Autodesk Inventor part; units mm, degrees
ref_plane "YZ Plane" through (0, 0, 0) normal (1, 0, 0) x (0, 1, 0)
ref_plane "XZ Plane" through (0, 0, 0) normal (0, 1, 0) x (-1, 0, 0)
ref_plane "XY Plane" through (0, 0, 0) normal (0, 0, 1) x (1, 0, 0)
ref_plane "РабПлоскость1" through (-34.9448, 28.465, -130.3508) normal (0, 0, 1) x (1, 0, 0)
ref_plane "РабПлоскость2" through (-162.802, 331.465, 111.3492) normal (0, 0, 1) x (1, 0, 0)
sketch "Эскиз1" plane through (-34.9448, 28.465, -130.3508) normal (0, 0, 1) x (1, 0, 0)
  line L0 (0, 3.6904) -> (-12.8571, 3.6904) construction
  line L1 (0, 3.6904) -> (0, 9.6905)
  line L2 (-12.8571, 9.6905) -> (0, 9.6905)
  line L3 (-12.8571, 3.6904) -> (-12.8571, 9.6905)
  line L4 (25.7143, 3.6904) -> (12.8571, 3.6904) construction
  line L5 (25.7143, 3.6904) -> (25.7143, 9.6905)
  line L6 (12.8571, 9.6905) -> (25.7143, 9.6905)
  line L7 (12.8571, 3.6904) -> (12.8571, 9.6905)
  line L8 (51.4286, 3.6904) -> (38.5714, 3.6904) construction
  line L9 (51.4286, 3.6904) -> (51.4286, 9.6905)
  line L10 (38.5714, 9.6905) -> (51.4286, 9.6905)
  line L11 (38.5714, 3.6904) -> (38.5714, 9.6905)
  line L12 (77.1429, 3.6904) -> (64.2857, 3.6904) construction
  line L13 (77.1429, 3.6904) -> (77.1429, 9.6905)
  line L14 (64.2857, 9.6905) -> (77.1429, 9.6905)
  line L15 (64.2857, 3.6904) -> (64.2857, 9.6905)
  line L16 (0, 3.6904) -> (12.8571, 3.6904)
  line L17 (25.7143, 3.6904) -> (38.5714, 3.6904)
  line L18 (51.4286, 3.6904) -> (64.2857, 3.6904)
  line L19 (-12.8571, 3.6904) -> (-12.8571, -50.3096)
  line L20 (-9.8571, -53.3096) -> (-4.7353, -53.3096)
  line L21 (77.1429, 3.6904) -> (77.1429, -50.3096)
  line L22 (74.1429, -53.3096) -> (69.021, -53.3096)
  line L23 (-1.8571, -53.3096) -> (66.1429, -53.3096) construction
  arc A0 (-1.7452, -56.0663) -> (66.0309, -56.0663) centre (32.1429, -53.3096) ccw
  arc A1 (-1.7452, -56.0663) -> (-4.7353, -53.3096) centre (-4.7353, -56.3096) ccw
  arc A2 (69.021, -53.3096) -> (66.0309, -56.0663) centre (69.021, -56.3096) ccw
  arc A3 (74.1429, -53.3096) -> (77.1429, -50.3096) centre (74.1429, -50.3096) ccw
  arc A4 (-12.8571, -50.3096) -> (-9.8571, -53.3096) centre (-9.8571, -50.3096) ccw
  circle A5 centre (32.1429, -53.3095) radius 2.375
  point P0 (34.9448, -28.465)
  point P1 (77.1429, -53.3096)
  dimension "d0" = 57
  dimension "d1" = 34
  dimension "d2" = 3
  dimension "d3" = 6
  dimension "d14" = 4.75
extrude "Выдавливание1" add sketch "Эскиз1" along normal blind 6
sketch "Эскиз2" plane through (-34.9448, 28.465, -130.3508) normal (0, 0, -1) x (-1, 0, 0)
  line L0 (-4.9286, 3.6904) -> (-4.9286, -2.6596)
  line L1 (-4.9286, -2.6596) -> (-3.6786, -2.6596)
  line L2 (-3.6786, -2.6596) -> (-3.6786, -4.9596)
  line L3 (-3.6786, -4.9596) -> (-4.9286, -4.9596)
  line L4 (-4.9286, -4.9596) -> (-4.9286, -11.3096)
  line L5 (-4.9286, -11.3096) -> (-7.9286, -11.3096)
  line L6 (-7.9286, -11.3096) -> (-7.9286, -4.9596)
  line L7 (-7.9286, -4.9596) -> (-9.1786, -4.9596)
  line L8 (-9.1786, -4.9596) -> (-9.1786, -2.6596)
  line L9 (-9.1786, -2.6596) -> (-7.9286, -2.6596)
  line L10 (-7.9286, -2.6596) -> (-7.9286, 3.6904)
  line L11 (-56.3571, 3.6904) -> (-59.3571, 3.6904)
  line L12 (-56.3571, 3.6904) -> (-56.3571, -2.6596)
  line L13 (-56.3571, -2.6596) -> (-55.1071, -2.6596)
  line L14 (-55.1071, -2.6596) -> (-55.1071, -4.9596)
  line L15 (-55.1071, -4.9596) -> (-56.3571, -4.9596)
  line L16 (-56.3571, -4.9596) -> (-56.3571, -11.3096)
  line L17 (-56.3571, -11.3096) -> (-59.3571, -11.3096)
  line L18 (-59.3571, -11.3096) -> (-59.3571, -4.9596)
  line L19 (-59.3571, -4.9596) -> (-60.6071, -4.9596)
  line L20 (-60.6071, -4.9596) -> (-60.6071, -2.6596)
  line L21 (-60.6071, -2.6596) -> (-59.3571, -2.6596)
  line L22 (-59.3571, -2.6596) -> (-59.3571, 3.6904)
  line L23 (-56.3571, 3.6904) -> (-59.3571, 3.6904)
  line L24 (-4.9286, 3.6904) -> (-7.9286, 3.6904)
  point P0 (-34.9448, -28.465)
  point P1 (-6.4286, 0)
  dimension "d9" = 5.5
  dimension "d10" = 2.3
  dimension "d11" = 15
extrude "Выдавливание2" cut sketch "Эскиз2" against normal blind 6
equation "\"d4\" = d3"
equation "\"d12\" = d3"
properties part number "Korpus 4"
Design review of the part built by this model. Coordinates are the model's own, in mm. A direction names the side the tool comes from. Give positions to 0.01 mm unless a question says otherwise; leave off trailing zeros. Loops run counter-clockwise (first coordinate to the right, second up) from the corner with the lowest first, then second, coordinate; pieces in that order, holes last. Notation, with made-up numbers: (53.5, 25.25) - (81.5, 25.25) arc R16 cw to (81.5, 42.25) - close; hole circle Ø1 at (-40, -1). An arc over 180 degrees is marked (long way). Use CSV: the item, a comma, the result in double quotes. Start each with the question number.
1. Draft analysis for pull direction X (two halves, no side actions). For faces 3 (the flat face through (-27.016, 20, -127)), 4 (the cylindrical face through (-37.67, -25.62, -127.39)), 5 (the cylindrical face through (32.02, -25.66, -127.39)), 6 (the flat face through (37, -24.845, -127)), state which applies: released by +X, released by -X, zero draft, split by the parting line, or undercut.
2. Wall thickness on L1, parallel to X at y = -27.5, z = -126.15; L2, parallel to Y at x = 35, z = -125.9; L3, parallel to X at y = -22, z = -128.2: over which ranges is each line inside the solid? List them lowest first.
3. Insertion check: P1, Ø3, axis at x = 0, z = -126, coming from the +Y side; P2, Ø1.5, axis at y = -36, z = -126, coming from the -X side. Each pin has a flat end and moves straight along its axis. Give the tip position at first contact, or say it passes through.
4. Machinability: for faces 1 (the flat face through (-25, 32.155, -127)), 2 (the flat face through (-47.802, 9, -127)), which of the approach directions +Z, -Z, +X, -X, +Y, -Y give a long, thin tool a straight path to every point of the face, cutting with its end or side? Answer none if there is none.
5. Add section A-A (y = 29). State the section outline as (x, z) points, plus the area to 3 significant figures.
6. Add section B-B (y = -41). State the section outline as (x, z) points, plus the area to 3 significant figures.
Results found:
1,face 3,"undercut"
1,face 4,"released by -X"
1,face 5,"released by +X"
1,face 6,"zero draft"
2,L1,"x = -36.7 to 31.1"
2,L2,"y = -24.84 to 38.16"
2,L3,"x = -47.8 to 42.19"
3,P1,"stops at y = 32.16"
3,P2,"stops at x = -35.17"
4,face 1,"+Z, -Z, +Y"
4,face 2,"+Z, -Z, -X, +Y, -Y"
5,outline,"(-47.8, -130.35) - (-30.02, -130.35) - (-30.02, -124.35) - (-47.8, -124.35) - close; (-27.02, -130.35) - (21.41, -130.35) - (21.41, -124.35) - (-27.02, -124.35) - close; (24.41, -130.35) - (42.2, -130.35) - (42.2, -124.35) - (24.41, -124.35) - close"
5,area,"504 mm²"
6,outline,"(-32.72, -130.35) - (27.11, -130.35) - (27.11, -124.35) - (-32.72, -124.35) - close"
6,area,"359 mm²"
